from build123d import *

# Parameters (mm, degrees)
SKETCH1_W           = 200
SKETCH1_H           = 100
SKETCH1_W_2         = 177
SKETCH1_H_2         = 80
BOSS_EXTRUDE1_DEPTH = 14
SKETCH2_W           = 200
SKETCH2_H           = 100
SKETCH2_W_2         = 184
SKETCH2_H_2         = 85
BOSS_EXTRUDE2_DEPTH = 13
SKETCH4_W           = 10.8
SKETCH4_H           = 13
CUT_EXTRUDE2_DEPTH  = 137.938854968
SKETCH5_W           = 8
SKETCH5_H           = 13
SKETCH5_H_2         = 21
CUT_EXTRUDE3_DEPTH  = 11
SKETCH7_W           = 1.4
SKETCH7_H           = 8
BOSS_EXTRUDE3_DEPTH = 11
SKETCH8_W           = 2.6
SKETCH8_H           = 8
BOSS_EXTRUDE4_DEPTH = 2
CHAMFER3_SIZE       = 2
CHAMFER4_SIZE       = 1.154700538
CHAMFER4_SIZE_2     = 2
MIRROR2_START       = 14.3
MIRROR2_DEPTH       = 8


# Read off the part's stored shape, not the designer's step: Mirror2
with BuildPart() as part:
    # Sketch1 → Boss-Extrude1 (new body)
    with BuildSketch(Plane.YZ):
        Rectangle(SKETCH1_W, SKETCH1_H)
        Rectangle(SKETCH1_W_2, SKETCH1_H_2, mode=Mode.SUBTRACT)
    extrude(amount=BOSS_EXTRUDE1_DEPTH)

    # Sketch2 → Boss-Extrude2 (add)
    with BuildSketch(Plane(origin=(0, 0, 0), x_dir=(0, -1, 0), z_dir=(-1, 0, 0))):
        Rectangle(SKETCH2_W, SKETCH2_H)
        Rectangle(SKETCH2_W_2, SKETCH2_H_2, mode=Mode.SUBTRACT)
    extrude(amount=BOSS_EXTRUDE2_DEPTH)

    # Sketch4 → Cut-Extrude2 (cut, through all)
    with BuildSketch(Plane.XY.offset(-42.5)):
        with Locations((-5.4, 79.5)):
            Rectangle(SKETCH4_W, SKETCH4_H)
        with Locations((-5.4, 26.5)):
            Rectangle(SKETCH4_W, SKETCH4_H)
        with Locations((-5.4, -26.5)):
            Rectangle(SKETCH4_W, SKETCH4_H)
        with Locations((-5.4, -79.5)):
            Rectangle(SKETCH4_W, SKETCH4_H)
    extrude(amount=-CUT_EXTRUDE2_DEPTH, mode=Mode.SUBTRACT)

    # Sketch5 → Cut-Extrude3 (cut)
    with BuildSketch(Plane(origin=(-13, 0, 0), x_dir=(0, -1, 0), z_dir=(-1, 0, 0))):
        with Locations((-96, 18.3)):
            Rectangle(SKETCH5_W, SKETCH5_H)
        with Locations((96, 22.3)):
            Rectangle(SKETCH5_W, SKETCH5_H_2)
    extrude(amount=-CUT_EXTRUDE3_DEPTH, mode=Mode.SUBTRACT)

    # Sketch7 → Boss-Extrude3 (add)
    with BuildSketch(Plane(origin=(-2, 0, 0), x_dir=(0, -1, 0), z_dir=(-1, 0, 0))):
        with Locations((-99.3, 18.3)):
            Rectangle(SKETCH7_W, SKETCH7_H)
        with Locations((99.3, 18.3)):
            Rectangle(SKETCH7_W, SKETCH7_H)
    extrude(amount=BOSS_EXTRUDE3_DEPTH)

    # Sketch8 → Boss-Extrude4 (add)
    with BuildSketch(Plane.XZ.offset(-98.6)):
        with Locations((-11.7, 18.3)):
            Rectangle(SKETCH8_W, SKETCH8_H)
    extrude(amount=BOSS_EXTRUDE4_DEPTH)

    # Chamfer3
    chamfer3_edges = [part.edges().sort_by_distance(p)[0] for p in [
        (-13, 96.6, 18.3),
    ]]
    chamfer(chamfer3_edges, length=CHAMFER3_SIZE)

    # Chamfer4
    # the kernel refuses this chamfer: 2, 1.154700538 mm, written as the material it takes off along each edge
    with BuildSketch(Plane(origin=(-10.4, 96.6, 27.474171509), x_dir=(-0.9983227437537927, -0.057893862402668146, 0), z_dir=(0, 0, -1))) as chamfer4_piece_1_section:
        Polygon((CHAMFER4_SIZE * 0.998322744082, CHAMFER4_SIZE * 0.0578938624217), (-CHAMFER4_SIZE_2 * 0.0578938624027, CHAMFER4_SIZE_2 * 0.998322743754), (0, 0), align=None)
    chamfer4_piece_1 = extrude(amount=18.348343019, mode=Mode.PRIVATE)
    chamfer4_piece_1 = split(chamfer4_piece_1, bisect_by=Plane(origin=(-10.737181007, 97.317358716, 24.8), z_dir=(0, 0, -1)), keep=Keep.TOP, mode=Mode.PRIVATE)
    chamfer4_piece_1 = split(chamfer4_piece_1, bisect_by=Plane(origin=(-10.737181007, 97.317358716, 11.8), z_dir=(0, 0, 1)), keep=Keep.TOP, mode=Mode.PRIVATE)
    add(chamfer4_piece_1, mode=Mode.SUBTRACT)

    # Mirror2 outline → Mirror2 (add)
    with BuildSketch(Plane.XY.offset(MIRROR2_START)):
        Polygon((-13, -98.6), (-10.4, -98.6), (-10.4, -97.754700538), (-11.512435565, -97.112435565), align=None)
    extrude(amount=MIRROR2_DEPTH)


solid = part.part
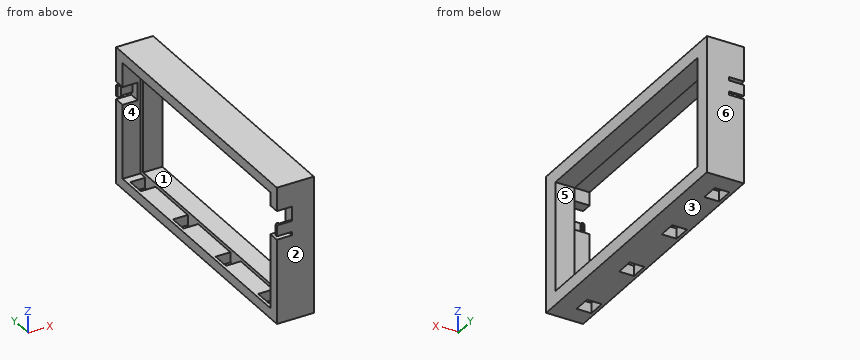
Can you work these out from the model? Positions are in its coordinate system, mm. Face numbers are marked on the shaded views. A direction names the side the tool comes from. Coordinates: 2 decimals unless noted, no trailing zeros. Write each loop counter-clockwise with the first axis right and the second up, starting at its lowest first coordinate (ties: lowest second). Pieces come first, ordered by that corner, then holes. Notation, with made-up numbers: (-3.5, 76.5) -> (21.5, 76.5) arc R26 cw to (21.5, 101.5) -> close; hole circle Ø3 at (18.25, 64.5). An arc over 180 degrees is marked (long way). Write item = value, one per line.
(1) Imagine slicing it at C-C (z = -16). Please give me the cut outline in (x, y).
Verdict:
outline = (-13, -100) -> (14, -100) -> (14, -88.5) -> (0, -88.5) -> (0, -92) -> (-13, -92) -> close; (-13, 92) -> (0, 92) -> (0, 88.5) -> (14, 88.5) -> (14, 100) -> (-13, 100) -> close
(2) Thinking about a two-plate mould opening in Y: for the marked faces 1, 2 and 3, which applies, +Y half, -Y half, draft (parallel to the pull), parting line (faces both ways), or undercut?
Verdict:
face_1 = undercut
face_2 = -Y half
face_3 = draft
(3) Imagine slicing it at D-D (x = -6.5). State how many separate pieces and enclosed holes the cut face has, and give its area (3 significant figures).
Verdict:
separate_pieces = 8
enclosed_holes = 0
area = 3,720 mm^2
(4) Imagine slicing it at B-B (y = -25). Please give me the cut outline in (x, z), and give its area (3 significant figures).
Verdict:
outline = (-13, -50) -> (-10.8, -50) -> (-10.8, -42.5) -> (-13, -42.5) -> close; (-13, 42.5) -> (0, 42.5) -> (0, 40) -> (14, 40) -> (14, 50) -> (-13, 50) -> close; (0, -50) -> (14, -50) -> (14, -40) -> (0, -40) -> close
area = 394 mm^2
(5) Imagine slicing it at A-A (x = 5). Please give me the cut outline in (y, z), and give its area (3 significant figures).
Verdict:
outline = (-100, -50) -> (100, -50) -> (100, 50) -> (-100, 50) -> close; hole (-88.5, -40) -> (88.5, -40) -> (88.5, 40) -> (-88.5, 40) -> close
area = 5,840 mm^2
(6) On a 3-axis mill with a long thin cutter (end or side, diameter ignored), from which of +Z, -Z, +X, -X, +Y, -Y can I reach the whole of each face in a straight line? I mean the marked faces 4, 5 and 6. Say none if no direction works.
Verdict:
face_4 = -X
face_5 = +X, -X
face_6 = +Z, -Z, +X, -X, +Y
(7) If I drill on probe 1 along Y at (x, z) = (-7.25, -43.5); probe 2 along Z at (x, y) = (6.5, -29); probe 3 along Y at (x, z) = (8.5, -32), over which ranges is the centre line in solid material (lowest first)?
Verdict:
probe_1 = -100 to -86, -73 to -33, -20 to 20, 33 to 73, 86 to 100
probe_2 = -50 to -40, 40 to 50
probe_3 = -100 to -88.5, 88.5 to 100
